```python
from build123d import *

# Parameters (mm, degrees)
F1_DEPTH = 50.8
F2_W     = 20.828
F2_H     = 38.1
F3_DEPTH = 50.8
F4_W     = 22.225
F4_H     = 53.975
F5_DEPTH = 50.8
F6_R     = 8.89
F7_R     = 2.54


with BuildPart() as f1:
    # F0 (on Top) → F1 (new body)
    with BuildSketch(Plane.XY):
        with BuildLine():
            ThreePointArc((-111.331622, 89), (-115.642145, 87.214523), (-117.427622, 82.904))
            Line((-117.427622, 82.904), (-117.427622, -82.904))
            ThreePointArc((-117.427622, -82.904), (-115.642145, -87.214523), (-111.331622, -89))
            Line((-111.331622, -89), (111.331622, -89))
            ThreePointArc((111.331622, -89), (115.642145, -87.214523), (117.427622, -82.904))
            Line((117.427622, -82.904), (117.427622, 82.904))
            ThreePointArc((117.427622, 82.904), (115.642145, 87.214523), (111.331622, 89))
            Line((111.331622, 89), (-111.331622, 89))
        make_face()
        with BuildLine():
            ThreePointArc((-60.918022, -10.802655), (-61.609639, -0.559986), (-60.913995, 9.68241))
            Line((-60.913995, 9.68241), (-55.212554, 14.261207))
            ThreePointArc((-55.212554, 14.261207), (-45.748511, 39.77658), (-28.391702, 60.737103))
            Line((-28.391702, 60.737103), (-27.407633, 67.742944))
            ThreePointArc((-27.407633, 67.742944), (-18.790824, 73.526894), (-9.485241, 78.121416))
            Line((-9.485241, 78.121416), (-2.738388, 75.428307))
            ThreePointArc((-2.738388, 75.428307), (24.098624, 80.048241), (50.935831, 75.42944))
            Line((50.935831, 75.42944), (57.610091, 78.186609))
            ThreePointArc((57.610091, 78.186609), (66.892407, 73.605247), (75.516596, 67.880422))
            Line((75.516596, 67.880422), (76.520517, 60.753405))
            ThreePointArc((76.520517, 60.753405), (79.783196, 57.954312), (82.843276, 54.935057))
            ThreePointArc((82.843276, 54.935057), (104.449894, 47.071779), (100.407804, 24.436881))
            ThreePointArc((100.407804, 24.436881), (101.514269, 20.155202), (102.319921, 15.806873))
            Line((102.319921, 15.806873), (108.049072, 10.873495))
            ThreePointArc((108.049072, 10.873495), (108.709842, 0.589153), (108.105719, -9.698672))
            Line((108.105719, -9.698672), (102.348457, -13.775574))
            ThreePointArc((102.348457, -13.775574), (92.855411, -39.306001), (75.46826, -60.272823))
            Line((75.46826, -60.272823), (74.544008, -67.341163))
            ThreePointArc((74.544008, -67.341163), (66.082602, -73.324939), (56.891661, -78.113213))
            Line((56.891661, -78.113213), (50.250983, -75.428069))
            ThreePointArc((50.250983, -75.428069), (23.341097, -80.124901), (-3.581639, -75.502299))
            Line((-3.581639, -75.502299), (-10.28992, -78.054152))
            ThreePointArc((-10.28992, -78.054152), (-19.562426, -73.562391), (-28.115124, -67.817248))
            Line((-28.115124, -67.817248), (-29.074377, -60.66791))
            ThreePointArc((-29.074377, -60.66791), (-32.330068, -57.869325), (-35.398386, -54.86649))
            ThreePointArc((-35.398386, -54.86649), (-59.811696, -48.379935), (-53.325141, -23.966625))
            ThreePointArc((-53.325141, -23.966625), (-54.434448, -19.687429), (-55.222977, -15.337682))
            Line((-55.222977, -15.337682), (-60.918022, -10.802655))
        make_face(mode=Mode.SUBTRACT)
    extrude(amount=F1_DEPTH)

    # F2 (on face) → F3 (cut)
    with BuildSketch(Plane.XY.offset(50.8)):
        with Locations((-94.313622, -57.25)):
            Rectangle(F2_W, F2_H)
        with Locations((-94.313622, -6.45)):
            Rectangle(F2_W, F2_H)
    extrude(amount=-F3_DEPTH, mode=Mode.SUBTRACT)

    # F4 (on face) → F5 (cut)
    with BuildSketch(Plane.XY.offset(50.8)):
        with Locations((-93.615122, 49.3125)):
            Rectangle(F4_W, F4_H)
    extrude(amount=-F5_DEPTH, mode=Mode.SUBTRACT)

    # F6
    f6_edges = [f1.edges().sort_by_distance(p)[0] for p in [
        (-104.727622, 12.6, 25.4),
        (-104.727622, -38.2, 25.4),
        (-104.727622, -25.5, 25.4),
        (-104.727622, -76.3, 25.4),
    ]]
    fillet(f6_edges, radius=F6_R)

    # F7
    f7_edges = [f1.edges().sort_by_distance(p)[0] for p in [
        (-82.502622, 76.3, 25.4),
        (-104.727622, 76.3, 25.4),
        (-82.502622, 22.325, 25.4),
        (-104.727622, 22.325, 25.4),
    ]]
    fillet(f7_edges, radius=F7_R)


solid = f1.part
```
Could you check a few things on this model? Use its own coordinates, in mm. A direction names the side the tool comes from. Round coordinates to 2 decimals unless told otherwise and drop trailing zeros. Loops run counter-clockwise (first coordinate to the right, second up) from the corner with the lowest first, then second, coordinate; pieces in that order, holes last. Notation, with made-up numbers: (39, -38) -> (68, -38) arc R25 ccw to (68, -21) -> close; hole circle Ø4 at (-37, 41). An arc over 180 degrees is marked (long way). One line per question, with ' | ' between items.
(1) If we section it at C-C on x = -49: List the corners of the cut face in (y, z) for me, and give its area (3 significant figures).
Model answer:
outline: (-89, 0) -> (-56.67, 0) -> (-56.67, 50.8) -> (-89, 50.8) -> close; (33.53, 0) -> (89, 0) -> (89, 50.8) -> (33.53, 50.8) -> close | area: 4,460 mm^2
(2) If we section it at D-D on z = 30: Count the separate pieces of the cut face and the enclosed holes in it, and give its area (3 significant figures).
Model answer:
separate pieces: 1 | enclosed holes: 4 | area: 17,300 mm^2
(3) If I drill on probe 1 along X at (y, z) = (-1.5, 11); probe 2 along Y at (x, z) = (-101, 35.5) (3 decimals); probe 3 along X at (y, z) = (-44, 39), over which ranges is the centre line in solid material (lowest first)?
Model answer:
probe 1: x = -117.43 to -104.73, -83.9 to -61.6, 108.69 to 117.43 | probe 2: y = -89 to -74.648, -39.852 to -23.848, 10.948 to 22.325, 76.3 to 89 | probe 3: x = -117.43 to -104.17, -83.9 to -61.63, 89.92 to 117.43
(4) If we section it at B-B on y = -51.5: List the corners of the cut face in (x, z) for me, and give its area (3 significant figures).
Model answer:
outline: (-117.43, 0) -> (-104.73, 0) -> (-104.73, 50.8) -> (-117.43, 50.8) -> close; (-83.9, 0) -> (-57.52, 0) -> (-57.52, 50.8) -> (-83.9, 50.8) -> close; (84.22, 0) -> (117.43, 0) -> (117.43, 50.8) -> (84.22, 50.8) -> close | area: 3,670 mm^2
(5) If we section it at A-A on x = 5: List the corners of the cut face in (y, z) for me, and give its area (3 significant figures).
Model answer:
outline: (-89, 0) -> (-78.02, 0) -> (-78.02, 50.8) -> (-89, 50.8) -> close; (77.74, 0) -> (89, 0) -> (89, 50.8) -> (77.74, 50.8) -> close | area: 1,130 mm^2
(6) Thinking about a two-plate mould opening in Y: for faces 3 (the face through (-117.428, 1, 25)), 4 (the face through (-90, 12.6, 26)), 5 (the face through (-104.728, -57, 26)), 6 (the face through (2, 89, 25)), which applies, released by +Y, released by -Y, zero draft, split by the parting line, or undercut?
Model answer:
face 3: zero draft | face 4: undercut | face 5: undercut | face 6: released by +Y
(7) For faces 1 (the face through (-115.689, -87.167, 25.044)), 2 (the face through (108.71, 0.73, 25.04)), which set-ups out of +Z, -Z, +X, -X, +Y, -Y let a thin tool reach every point of the face, with its end or its side?
Model answer:
face 1: +Z, -Z, -X, -Y | face 2: +Z, -Z
